```python
from build123d import *

# Parameters (mm, degrees)
SCHIZZO1_W                             = 90
SCHIZZO1_H                             = 150
ESTRUSIONE_ESTRUSIONE1_DEPTH           = 90
SCHIZZO4_W                             = 60
SCHIZZO4_H                             = 70
TAGLIO_ESTRUSIONE2_DEPTH               = 90
RACCORDO5_R                            = 45
RACCORDO6_R                            = 45
SMUSSO2_SIZE                           = 20
SCHIZZO7_W                             = 50
SCHIZZO7_H                             = 44.753189799
ESTRUSIONE_ESTRUSIONE2_DEPTH           = 50
SMUSSO3_SIZE                           = 20
SMUSSO3_SIZE2                          = 34.641016151
RACCORDO7_R                            = 10
RACCORDO8_R                            = 10
SCHIZZO9_W                             = 50
SCHIZZO9_H                             = 50
ESTRUSIONE_ESTRUSIONE3_DEPTH           = 5
RACCORDO9_R                            = 10
SCHIZZO13_W                            = 45
SCHIZZO13_H                            = 38.415996799
TAGLIO_ESTRUSIONE3_DEPTH               = 79.978264331
SCHIZZO14_W                            = 117.844501366
SCHIZZO14_H                            = 59.041021869
TAGLIO_ESTRUSIONE4_DEPTH               = 8
SCHIZZO18_R                            = 5
TAGLIO_ESTRUSIONE5_DEPTH               = 9
SCHIZZO16_W                            = 4
SCHIZZO16_H                            = 20
TAGLIO_ESTRUSIONE7_DEPTH               = 2
SCHIZZO23_W                            = 76
SCHIZZO23_H                            = 117.844501366
TAGLIO_ESTRUSIONE8_DEPTH               = 38
FORO_PER_VITE_M2_2_D                   = 2.4
FORO_PER_VITE_M2_2_DEPTH               = 4
FORO_PER_VITE_M4_1_D                   = 4.5
FORO_PER_VITE_M4_1_DEPTH               = 10
SCHIZZO29_W                            = 60
SCHIZZO29_H                            = 11.209863528
TAGLIO_ESTRUSIONE9_DEPTH               = 30
SCHIZZO36_W                            = 46.07976418
SCHIZZO36_H                            = 28.262497783
TAGLIO_ESTRUSIONE12_DEPTH              = 28
ESTRUSIONE_ESTRUSIONE4_REACH           = 170.388
SCHIZZO38_R                            = 6
SCHIZZO38_R_2                          = 2.5
TAGLIO_ESTRUSIONE13_DEPTH              = 28
SCHIZZO39_R                            = 9
SCHIZZO39_W                            = 10
SCHIZZO39_H                            = 10
TAGLIO_ESTRUSIONE14_DEPTH              = 2
SCHIZZO40_W                            = 32
SCHIZZO40_H                            = 10
TAGLIO_ESTRUSIONE15_DEPTH              = 10
SCHIZZO42_R                            = 4
TAGLIO_ESTRUSIONE16_DEPTH              = 3
FORO_SVASATO_PER_VITE_M2_3_D           = 2.4
FORO_SVASATO_PER_VITE_M2_3_DEPTH       = 6
FORO_SVASATO_PER_VITE_M2_3_CSINK_D     = 4.4
FORO_SVASATO_PER_VITE_M2_3_CSINK_ANGLE = 90
FORO_SVASATO_PER_VITE_M2_3_TIP         = 0.721032743
SCHIZZO53_R                            = 9
TAGLIO_ESTRUSIONE19_DEPTH              = 2.75
SCHIZZO54_W                            = 60
SCHIZZO54_H                            = 36.634637838
TAGLIO_ESTRUSIONE20_DEPTH              = 24.75
SCHIZZO55_W                            = 50
SCHIZZO55_H                            = 69.198351347
TAGLIO_ESTRUSIONE21_DEPTH              = 66
SCHIZZO57_W                            = 18.365362162
SCHIZZO57_H                            = 38.415996799
ESTRUSIONE_ESTRUSIONE5_DEPTH           = 47
SCHIZZO58_W                            = 7
SCHIZZO58_H                            = 32
ESTRUSIONE_ESTRUSIONE6_DEPTH           = 11


with BuildPart() as part:
    # Schizzo1 → Estrusione-Estrusione1 (new body)
    with BuildSketch(Plane(origin=(0, 0, 0), x_dir=(1, 0, 0), z_dir=(0, 1, 0))):
        Rectangle(SCHIZZO1_W, SCHIZZO1_H)
    extrude(amount=ESTRUSIONE_ESTRUSIONE1_DEPTH)

    # Schizzo4 → Taglio-Estrusione2 (cut)
    with BuildSketch(Plane(origin=(0, 90, 0), x_dir=(1, 0, 0), z_dir=(0, 1, 0))):
        with Locations((0, 15)):
            Rectangle(SCHIZZO4_W, SCHIZZO4_H)
    extrude(amount=-TAGLIO_ESTRUSIONE2_DEPTH, mode=Mode.SUBTRACT)

    # Raccordo5
    # the kernel refuses this fillet: 45 mm, written as the material it takes off along each edge
    with BuildSketch(Plane(origin=(-45, 90, -187.5), x_dir=(0, -1, 0), z_dir=(0, 0, 1))) as raccordo5_piece_1:
        with BuildLine():
            CenterArc((RACCORDO5_R, RACCORDO5_R), RACCORDO5_R, 180, 90)
            Line((0, RACCORDO5_R), (0, 0))
            Line((0, 0), (RACCORDO5_R, 0))
        make_face()
    extrude(amount=375, mode=Mode.SUBTRACT)

    # Raccordo6
    # the kernel refuses this fillet: 45 mm, written as the material it takes off along each edge
    with BuildSketch(Plane(origin=(45, 90, 187.5), x_dir=(0, -1, 0), z_dir=(0, 0, -1))) as raccordo6_piece_1:
        with BuildLine():
            CenterArc((RACCORDO6_R, RACCORDO6_R), RACCORDO6_R, 180, 90)
            Line((0, RACCORDO6_R), (0, 0))
            Line((0, 0), (RACCORDO6_R, 0))
        make_face()
    extrude(amount=375, mode=Mode.SUBTRACT)

    # Smusso2
    smusso2_edges = [part.edges().sort_by_distance(p)[0] for p in [
        (-45, 22.5, 75),
        (0, 90, 75),
        (45, 22.5, 75),
        (0, 90, 75),
    ]]
    chamfer(smusso2_edges, length=SMUSSO2_SIZE)

    # Schizzo7 → Estrusione-Estrusione2 (add)
    with BuildSketch(Plane.XY.offset(75)):
        with Locations((0, 22.3765949)):
            Rectangle(SCHIZZO7_W, SCHIZZO7_H)
    extrude(amount=ESTRUSIONE_ESTRUSIONE2_DEPTH)

    # Smusso3
    smusso3_edges = [part.edges().sort_by_distance(p)[0] for p in [
        (0, 44.753189799, 125),
    ]]
    smusso3_side = [part.faces().sort_by_distance(p)[0] for p in [
        (0, 44.753189799, 100),
    ]]
    chamfer(smusso3_edges, length=SMUSSO3_SIZE, length2=SMUSSO3_SIZE2, reference=smusso3_side[0])

    # Raccordo7
    raccordo7_edges = [part.edges().sort_by_distance(p)[0] for p in [
        (0, 44.753189799, 105),
    ]]
    fillet(raccordo7_edges, radius=RACCORDO7_R)

    # Raccordo8
    raccordo8_edges = [part.edges().sort_by_distance(p)[0] for p in [
        (0, 10.112173648, 125),
    ]]
    fillet(raccordo8_edges, radius=RACCORDO8_R)

    # Schizzo9 → Estrusione-Estrusione3 (add)
    with BuildSketch(Plane.XZ):
        with Locations((0, 100)):
            Rectangle(SCHIZZO9_W, SCHIZZO9_H)
    extrude(amount=ESTRUSIONE_ESTRUSIONE3_DEPTH)

    # Raccordo9
    raccordo9_edges = [part.edges().sort_by_distance(p)[0] for p in [
        (-45, 22.5, -75),
        (0, 90, -75),
        (45, 22.5, -75),
        (0, 90, -75),
    ]]
    fillet(raccordo9_edges, radius=RACCORDO9_R)

    # Schizzo13 → Taglio-Estrusione3 (cut)
    with BuildSketch(Plane(origin=(0, 0, 20), x_dir=(-1, 0, 0), z_dir=(0, 0, -1))):
        with Locations((0, 19.2079984)):
            Rectangle(SCHIZZO13_W, SCHIZZO13_H)
    extrude(amount=-TAGLIO_ESTRUSIONE3_DEPTH, mode=Mode.SUBTRACT)

    # Schizzo14 → Taglio-Estrusione4 (cut)
    with BuildSketch(Plane.ZY.offset(-30)):
        with Locations((-2.287612845, 29.520510935)):
            Rectangle(SCHIZZO14_W, SCHIZZO14_H)
    taglio_estrusione4 = extrude(amount=-TAGLIO_ESTRUSIONE4_DEPTH, mode=Mode.SUBTRACT)

    # Specchia1: Taglio-Estrusione4 across plane
    add(taglio_estrusione4.mirror(Plane(origin=(0, 0, 0), x_dir=(0, 0, 1), z_dir=(1, 0, 0))), mode=Mode.SUBTRACT)

    # Schizzo18 → Taglio-Estrusione5 (cut)
    with BuildSketch(Plane.ZY.offset(-30)):
        with Locations((-15, 48.541019662)):
            Circle(SCHIZZO18_R)
    extrude(amount=-TAGLIO_ESTRUSIONE5_DEPTH, mode=Mode.SUBTRACT)

    # Schizzo16 → Taglio-Estrusione7 (cut)
    with BuildSketch(Plane.XZ.offset(-59.041021869)):
        with Locations((32, -15)):
            Rectangle(SCHIZZO16_W, SCHIZZO16_H)
    extrude(amount=-TAGLIO_ESTRUSIONE7_DEPTH, mode=Mode.SUBTRACT)

    # Schizzo23 → Taglio-Estrusione8 (cut)
    with BuildSketch(Plane.XZ):
        with Locations((0, -2.287612845)):
            Rectangle(SCHIZZO23_W, SCHIZZO23_H)
    extrude(amount=-TAGLIO_ESTRUSIONE8_DEPTH, mode=Mode.SUBTRACT)

    # Foro per Vite M2-2
    with Locations(Plane(origin=(0, 0, 0), x_dir=(-1, 0, 0), z_dir=(0, -1, 0))):
        with Locations((40, 67), (30, -61.514718626), (-30, -61.514718626), (-40, 67), (-41.5, 5), (41.5, 5)):
            Hole(FORO_PER_VITE_M2_2_D / 2, depth=FORO_PER_VITE_M2_2_DEPTH)

    # Foro per Vite M4-1
    with Locations(Plane(origin=(0, -5, 84.779580177), x_dir=(0, 0, -1), z_dir=(0, -1, 0))):
        with Locations((0, 0)):
            Hole(FORO_PER_VITE_M4_1_D / 2, depth=FORO_PER_VITE_M4_1_DEPTH)

    # Schizzo29 → Taglio-Estrusione9 (cut)
    with BuildSketch(Plane.XZ.offset(-38)):
        with Locations((0, -55.604931764)):
            Rectangle(SCHIZZO29_W, SCHIZZO29_H)
    extrude(amount=-TAGLIO_ESTRUSIONE9_DEPTH, mode=Mode.SUBTRACT)

    # Schizzo36 → Taglio-Estrusione12 (cut)
    with BuildSketch(Plane(origin=(0, 56.654631148, 98.128699633), x_dir=(1, 0, 0), z_dir=(0, 0.5000000000000012, 0.8660254037844378))):
        with Locations((0, -35.289606117)):
            Rectangle(SCHIZZO36_W, SCHIZZO36_H)
    extrude(amount=-TAGLIO_ESTRUSIONE12_DEPTH, mode=Mode.SUBTRACT)

    # Schizzo37 → Estrusione-Estrusione4 (add, up to next)
    with BuildSketch(Plane.ZY.offset(-23.03988209), mode=Mode.PRIVATE) as estrusione_estrusione4_sk1:
        Polygon((122.839127138, 13.854915234), (108.707878246, 38.330956288), (106.809101084, 37.234696782), (120.940349975, 12.758655728), align=None)
    estrusione_estrusione4_tool1 = extrude(estrusione_estrusione4_sk1.sketch, amount=ESTRUSIONE_ESTRUSIONE4_REACH, mode=Mode.PRIVATE) - part.part
    add(estrusione_estrusione4_tool1.solids().sort_by_distance((23.039882, 25.544806, 114.824114))[0])

    # Schizzo38 → Taglio-Estrusione13 (cut)
    with BuildSketch(Plane(origin=(0, 56.654631148, 98.128699633), x_dir=(1, 0, 0), z_dir=(0, 0.5000000000000013, 0.8660254037844379))):
        with Locations(Location((-12.5, -35.289606117, 0), (0, 0, 270))):
            Circle(SCHIZZO38_R)
        with Locations(Location((12.5, -35.289606117, 0), (0, 0, 270))):
            Circle(SCHIZZO38_R_2)
    extrude(amount=-TAGLIO_ESTRUSIONE13_DEPTH, mode=Mode.SUBTRACT)

    # Schizzo39 → Taglio-Estrusione14 (cut)
    with BuildSketch(Plane(origin=(-38, 0, 0), x_dir=(0, 0, -1), z_dir=(1, 0, 0))):
        with Locations(Location((15, 48.541019662, 0), (0, 0, 90))):
            Circle(SCHIZZO39_R)
        with Locations((0, 48.541019662)):
            Rectangle(SCHIZZO39_W, SCHIZZO39_H)
        with Locations((30, 48.541019662)):
            Rectangle(SCHIZZO39_W, SCHIZZO39_H)
    extrude(amount=-TAGLIO_ESTRUSIONE14_DEPTH, mode=Mode.SUBTRACT)

    # Schizzo40 → Taglio-Estrusione15 (cut)
    with BuildSketch(Plane.ZY.offset(45)):
        with Locations((38, 10)):
            Rectangle(SCHIZZO40_W, SCHIZZO40_H)
    taglio_estrusione15 = extrude(amount=-TAGLIO_ESTRUSIONE15_DEPTH, mode=Mode.SUBTRACT)

    # Schizzo42 → Taglio-Estrusione16 (cut)
    with BuildSketch(Plane.ZY.offset(45)):
        with Locations((-30, 48.541019662)):
            Circle(SCHIZZO42_R)
        with Locations((0, 48.541019662)):
            Circle(SCHIZZO42_R)
    extrude(amount=-TAGLIO_ESTRUSIONE16_DEPTH, mode=Mode.SUBTRACT)

    # Foro svasato per Vite M2-3
    with Locations(Plane.ZY.offset(42)):
        with Locations((-30, 48.541019662), (0, 48.541019662)):
            CounterSinkHole(FORO_SVASATO_PER_VITE_M2_3_D / 2, FORO_SVASATO_PER_VITE_M2_3_CSINK_D / 2, depth=FORO_SVASATO_PER_VITE_M2_3_DEPTH, counter_sink_angle=FORO_SVASATO_PER_VITE_M2_3_CSINK_ANGLE)
            with Locations((0, 0, -(FORO_SVASATO_PER_VITE_M2_3_DEPTH + FORO_SVASATO_PER_VITE_M2_3_TIP / 2))):  # 118° drill point
                Cone(0, FORO_SVASATO_PER_VITE_M2_3_D / 2, FORO_SVASATO_PER_VITE_M2_3_TIP, mode=Mode.SUBTRACT)

    # Schizzo53 → Taglio-Estrusione19 (cut)
    with BuildSketch(Plane(origin=(-40, 0, 0), x_dir=(0, 0, -1), z_dir=(1, 0, 0))):
        with Locations(Location((15, 48.541019662, 0), (0, 0, 90))):
            Circle(SCHIZZO53_R)
    extrude(amount=-TAGLIO_ESTRUSIONE19_DEPTH, mode=Mode.SUBTRACT)

    # Schizzo54 → Taglio-Estrusione20 (cut)
    with BuildSketch(Plane.XZ.offset(-38)):
        with Locations((0, 38.317318919)):
            Rectangle(SCHIZZO54_W, SCHIZZO54_H)
    extrude(amount=-TAGLIO_ESTRUSIONE20_DEPTH, mode=Mode.SUBTRACT)

    # Schizzo55 → Taglio-Estrusione21 (cut)
    with BuildSketch(Plane(origin=(0, 44.753189799, 0), x_dir=(1, 0, 0), z_dir=(0, 1, 0))):
        with Locations((0, -109.599175673)):
            Rectangle(SCHIZZO55_W, SCHIZZO55_H)
    extrude(amount=-TAGLIO_ESTRUSIONE21_DEPTH, mode=Mode.SUBTRACT)

    # Schizzo57 → Estrusione-Estrusione5 (add)
    with BuildSketch(Plane(origin=(-22.5, 0, 0), x_dir=(0, 0, -1), z_dir=(1, 0, 0))):
        with Locations((-65.817318919, 19.2079984)):
            Rectangle(SCHIZZO57_W, SCHIZZO57_H)
    extrude(amount=ESTRUSIONE_ESTRUSIONE5_DEPTH)

    # Specchia2: Taglio-Estrusione15 across plane
    add(taglio_estrusione15.mirror(Plane(origin=(0, 0, 0), x_dir=(0, 0, 1), z_dir=(1, 0, 0))), mode=Mode.SUBTRACT)

    # Schizzo58 → Estrusione-Estrusione6 (add)
    with BuildSketch(Plane.XZ.offset(-15)):
        with Locations((-41.5, 38)):
            Rectangle(SCHIZZO58_W, SCHIZZO58_H)
    extrude(amount=ESTRUSIONE_ESTRUSIONE6_DEPTH)


solid = part.part
```
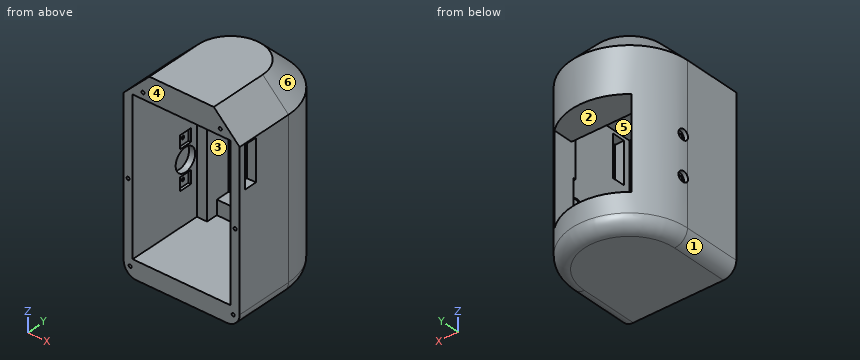
CAD build for the part. Positions are in the model's coordinates, mm. Face numbers are marked on the shaded views. A direction names the side the tool comes from. Round coordinates to 2 decimals unless told otherwise and drop trailing zeros. Loops run counter-clockwise (first coordinate to the right, second up) from the corner with the lowest first, then second, coordinate; pieces in that order, holes last. Notation, with made-up numbers: M 29.5,82.5 L 82.5,82.5 A31 ccw 82.5,119.5 Z; hole C 84,80.25 d10. An arc over 180 degrees is marked long. Use a Markdown table: item, result. Add a question column.
(1) Pull direction Z, two halves, no side cores. Call the marked faces 4, 5 and 6: +Z half, -Z half, draft (parallel to the pull), parting line (faces both ways), or undercut.
(2) Drill centre lines: line 1 (Z direction, x = -30, y = 1); line 2 (X direction, y = 9.5, z = -40); line 3 (Z direction, x = -8.5, y = 42). Where is each one in solid material? Low to high.
(3) Cut at A-A (z = 39). Give the cut face in (x, y), and give its area (3 significant figures).
(4) Cut at C-C (y = 12.5). Give the cut face in (x, z).
(5) Cut at B-B (x = 0). Give the cut face in (y, z).
(6) Flat gauge pins, fed straight in: pin 1 (1 mm diameter, centred on x = 22, y = 76.5, fed in from -Z); pin 2 (5 mm diameter, centred on y = 64.5, z = 8, fed in from -X); pin 3 (2 mm diameter, centred on x = 30, z = 61.51, fed in from -Y); pin 4 (10 mm diameter, centred on x = 16, z = 11.5, fed in from -Y). Where does each tip first touch, or does it go through?
(7) Cut at D-D (z = 18). Give the cut face in (x, y), and give its area (3 significant figures).
(8) Which spindle directions (+Z, -Z, +X, -X, +Y, -Y) get a long thin tool onto all of the face, cutting with end or side? Do the marked faces 1, 2 and 3. Say none if no direction does.
Geometry says:
| question | item | result |
|---|---|---|
| 1 | face 4 | draft |
| 1 | face 5 | undercut |
| 1 | face 6 | +Z half |
| 2 | line 1 | z = -75 to -61.21, 56.63 to 60.31, 62.71 to 70 |
| 2 | line 2 | x = -45 to -38, 38 to 45 |
| 2 | line 3 | z = -75 to -61.21, 56.63 to 75 |
| 3 | outline | M -45,0 L -38,0 L -38,59.04 L -30,59.04 L -30,62.75 L 30,62.75 L 30,59.04 L 38,59.04 L 38,15 L 45,15 L 45,45 A45 ccw -45,45 Z; M 38,0 L 45,0 L 45,5 L 38,5 Z |
| 3 | area | 2,450 mm² |
| 4 | outline | M -45,-65 A10 ccw -35,-75 L 35,-75 A10 ccw 45,-65 L 45,22 L 38,22 L 38,-61.21 L -38,-61.21 L -38,56.63 L 38,56.63 L 38,54 L 45,54 L 45,55 L 25,75 L -25,75 L -45,55 Z |
| 5 | outline | M 0,-75 L 80,-75 A10 ccw 90,-65 L 90,-50 L 68,-50 L 68,-61.21 L 0,-61.21 Z; M 0,56.63 L 62.75,56.63 L 62.75,20 L 90,20 L 90,55 L 70,75 L 0,75 Z |
| 6 | pin 1 | stops at z = -74.56 |
| 6 | pin 2 | stops at x = -41.67 |
| 6 | pin 3 | stops at y = 4 |
| 6 | pin 4 | passes through |
| 7 | outline | M -45,0 L -38,0 L -38,59.04 L -30,59.04 L -30,78.54 A45 ccw -45,45 Z; M 30,59.04 L 38,59.04 L 38,0 L 45,0 L 45,45 A45 ccw 30,78.54 Z |
| 7 | area | 1,100 mm² |
| 8 | face 1 | -Z, -X, +Y, -Y |
| 8 | face 2 | +Y, -Y |
| 8 | face 3 | -Y |
